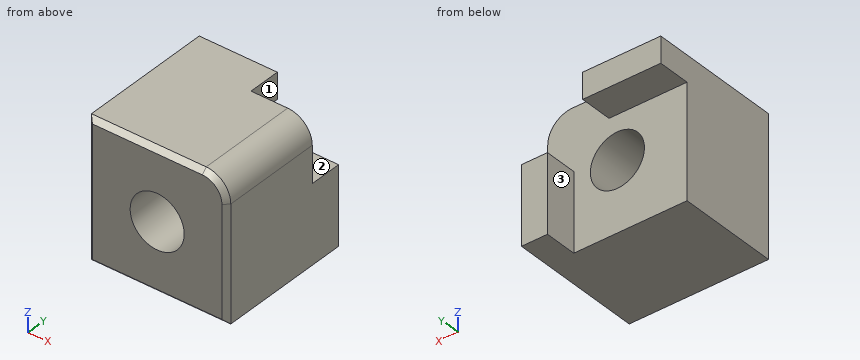
```python
from build123d import *

# Parameters (mm, degrees)
BASE_W              = 8.5
BASE_H              = 8.5
BOSS_EXTRUDE1_DEPTH = 8
CUTOUT_W            = 7
CUTOUT_H            = 7
CUT_EXTRUDE1_DEPTH  = 1.5
SKETCH3_W           = 1.5
SKETCH3_H           = 1.5
CUT_EXTRUDE2_DEPTH  = 12.448253142
FILLET3_R           = 0.508
FILLET4_R           = 1.5
M4_TAPPED_HOLE1_D   = 3.3
CHAMFER1_SIZE       = 0.3
CUT_EXTRUDE3_START  = -1.5
CUT_EXTRUDE3_DEPTH  = 1.5
SKETCH16_W          = 1.5875
SKETCH16_H          = 4.7625
SKETCH16_W_2        = 4.7625
SKETCH16_H_2        = 1.5875
BOSS_EXTRUDE2_DEPTH = 2


with BuildPart() as part:
    # Base → Boss-Extrude1 (new body)
    with BuildSketch(Plane(origin=(0, 0, 0), x_dir=(1, 0, 0), z_dir=(0, 1, 0))):
        Rectangle(BASE_W, BASE_H)
    extrude(amount=-BOSS_EXTRUDE1_DEPTH)

    # Cutout → Cut-Extrude1 (cut)
    with BuildSketch(Plane(origin=(0, 0, 0), x_dir=(1, 0, 0), z_dir=(0, 1, 0))):
        with Locations((-0.75, 0.75)):
            Rectangle(CUTOUT_W, CUTOUT_H)
    extrude(amount=-CUT_EXTRUDE1_DEPTH, mode=Mode.SUBTRACT)

    # Sketch3 → Cut-Extrude2 (cut, through all)
    with BuildSketch(Plane.ZY.offset(-2.75)):
        with Locations((-3.5, -0.75)):
            Rectangle(SKETCH3_W, SKETCH3_H)
    cut_extrude2 = extrude(amount=-CUT_EXTRUDE2_DEPTH, mode=Mode.SUBTRACT)

    # Mirror1: Cut-Extrude2 across plane
    add(cut_extrude2.mirror(Plane(origin=(0, 0, 0), x_dir=(0.7071067811865476, 0, 0.7071067811865475), z_dir=(0.7071067811865475, 0, -0.7071067811865476))), mode=Mode.SUBTRACT)

    # Fillet3
    fillet3_edges = [part.edges().sort_by_distance(p)[0] for p in [
        (2.75, -0.75, 2.75),
    ]]
    fillet(fillet3_edges, radius=FILLET3_R)

    # Fillet4
    fillet4_edges = [part.edges().sort_by_distance(p)[0] for p in [
        (4.25, -4, 4.25),
    ]]
    fillet(fillet4_edges, radius=FILLET4_R)

    # M4 Tapped Hole1 (through all)
    with Locations(Plane(origin=(0, -1.5, 0), x_dir=(1, 0, 0), z_dir=(0, 1, 0))):
        with Locations((0, 0)):
            Hole(M4_TAPPED_HOLE1_D / 2)

    # Chamfer1
    chamfer1_edges = [part.edges().sort_by_distance(p)[0] for p in [
        (-4.25, -8, 0),
        (-0.75, -8, 4.25),
        (4.25, -8, -0.75),
        (3.810660172, -8, 3.810660172),
        (0, -8, -4.25),
    ]]
    chamfer(chamfer1_edges, length=CHAMFER1_SIZE)

    # Sketch14 → Cut-Extrude3 (cut)
    with BuildSketch(Plane(origin=(0, 0, 0), x_dir=(1, 0, 0), z_dir=(0, 1, 0)).offset(CUT_EXTRUDE3_START)):
        with BuildLine():
            Line((-2.75, -4.25), (2.75, -4.25))
            ThreePointArc((2.75, -4.25), (3.810660172, -3.810660172), (4.25, -2.75))
            Line((4.25, -2.75), (4.25, 2.75))
            Line((4.25, 2.75), (2.75, 2.75))
            Line((2.75, 2.75), (2.75, -2.242))
            ThreePointArc((2.75, -2.242), (2.601210245, -2.601210245), (2.242, -2.75))
            Line((2.242, -2.75), (-2.75, -2.75))
            Line((-2.75, -2.75), (-2.75, -4.25))
        make_face()
    extrude(amount=CUT_EXTRUDE3_DEPTH, mode=Mode.SUBTRACT)

    # Sketch16 → Boss-Extrude2 (add)
    with BuildSketch(Plane(origin=(0, -1.5, 0), x_dir=(1, 0, 0), z_dir=(0, 1, 0))):
        with Locations((3.45625, 1.86875)):
            Rectangle(SKETCH16_W, SKETCH16_H)
        with Locations((-1.86875, -3.45625)):
            Rectangle(SKETCH16_W_2, SKETCH16_H_2)
    extrude(amount=BOSS_EXTRUDE2_DEPTH)


solid = part.part
```
For this review, take the finished solid that the model builds, in its own axes (mm). Face numbers are marked on the shaded views. A direction names the side the tool comes from. Round coordinates to 2 decimals unless told otherwise and drop trailing zeros. Write each loop counter-clockwise with the first axis right and the second up, starting at its lowest first coordinate (ties: lowest second). Pieces come first, ordered by that corner, then holes. Notation, with made-up numbers: (31.5, 5.25) -> (67.5, 5.25) arc R17 ccw to (67.5, 20.25) -> close; hole circle Ø7 at (50.25, 64). An arc over 180 degrees is marked (long way). One line per question, with ' | ' between items. Start each with the question number.
1) Add section B-B (z = 0). Write out the cut boundary in (x, y), and give its area (3 significant figures).
2) Wall thickness on line 1 along Z through (x, y) = (0, -3); line 2 along X through (y, z) = (-6.5, 0.25); line 3 along Y through (x, z) = (0.75, 3): over which ranges is each line inside the solid? List them lowest first.
3) Add section D-D (y = -1.75). Write out the cut boundary in (x, z).
4) Add section A-A (y = 0.25). Write out the cut boundary in (x, z).
5) Machinability: for the marked faces 1, 2 and 3, which of the approach directions +Z, -Z, +X, -X, +Y, -Y give a long, thin tool a straight path to every point of the face, cutting with its end or side? Answer none if there is none.
6) For pin 1 Ø4 at (x, y) = (1.5, -1) entering from -Z; pin 2 Ø2 at (y, z) = (0, -2) entering from -X; pin 3 Ø0.5 at (x, y) = (3, -0.5) entering from +Z; pin 4 Ø3 at (x, z) = (-3, -1.5) entering from +Y, all flat-tipped, find the tip position at first contact; note any pin that passes through.
7) Add section C-C (x = 0). Write out the cut boundary in (y, z), and give its area (3 significant figures).
Reported:
1) outline: (-4.25, -7.7) -> (-3.95, -8) -> (-1.65, -8) -> (-1.65, -1.5) -> (-4.25, -1.5) -> close; (1.65, -8) -> (3.95, -8) -> (4.25, -7.7) -> (4.25, 0.5) -> (2.66, 0.5) -> (2.66, -1.5) -> (1.65, -1.5) -> close | area: 36.9 mm²
2) line 1: z = -4.25 to -1.65, 1.65 to 4.25 | line 2: x = -4.25 to -1.63, 1.63 to 4.25 | line 3: y = -8 to -1.5
3) outline: (-4.25, -4.25) -> (4.25, -4.25) -> (4.25, 2.75) arc R1.5 ccw to (2.75, 4.25) -> (-4.25, 4.25) -> close; hole circle Ø3.3 at (0, 0)
4) outline: (-4.25, 2.66) -> (0.51, 2.66) -> (0.51, 4.25) -> (-4.25, 4.25) -> close; (2.66, -4.25) -> (4.25, -4.25) -> (4.25, 0.51) -> (2.66, 0.51) -> close
5) face 1: +Z, -Z, +X, +Y | face 2: +Z, +X, -X, +Y | face 3: +Z, -Z, -X, +Y
6) pin 1: stops at z = -4.25 | pin 2: stops at x = 2.66 | pin 3: stops at z = 0.51 | pin 4: stops at y = -1.5
7) outline: (-8, -3.95) -> (-7.7, -4.25) -> (-1.5, -4.25) -> (-1.5, -1.65) -> (-8, -1.65) -> close; (-8, 1.65) -> (-1.5, 1.65) -> (-1.5, 2.66) -> (0.5, 2.66) -> (0.5, 4.25) -> (-7.7, 4.25) -> (-8, 3.95) -> close | area: 36.9 mm²
